from build123d import *

# Parameters (mm, degrees)
SKETCH1_W                   = 228.6
SKETCH1_H                   = 139.7
SKETCH1_W_2                 = 203.2
SKETCH1_H_2                 = 114.3
BOSS_EXTRUDE1_DEPTH         = 6.35
BOSS_EXTRUDE2_DEPTH         = 6.35
FILLET1_R                   = 6.35
FILLET2_R                   = 6.35
F_1_4_CLEARANCE_HOLE1_D     = 6.7564
F_1_4_CLEARANCE_HOLE1_DEPTH = 9.906
F_1_4_CLEARANCE_HOLE1_TIP   = 2.029827343


with BuildPart() as part:
    # Sketch1 → Boss-Extrude1 (new body)
    with BuildSketch(Plane.XY):
        Rectangle(SKETCH1_W, SKETCH1_H)
        Rectangle(SKETCH1_W_2, SKETCH1_H_2, mode=Mode.SUBTRACT)
    extrude(amount=BOSS_EXTRUDE1_DEPTH)

    # Sketch2 → Boss-Extrude2 (add)
    with BuildSketch(Plane.XY.offset(6.35)):
        with BuildLine():
            Line((-96.930261692, 65.451756991), (0, 10.928484789))
            Line((0, 10.928484789), (96.930261692, 65.451756991))
            ThreePointArc((96.930261692, 65.451756991), (109.901756991, 61.819738308), (106.269738308, 48.848243009))
            Line((106.269738308, 48.848243009), (19.428417403, 0))
            Line((19.428417403, 0), (106.269738308, -48.848243009))
            ThreePointArc((106.269738308, -48.848243009), (109.901756991, -61.819738308), (96.930261692, -65.451756991))
            Line((96.930261692, -65.451756991), (0, -10.928484789))
            Line((0, -10.928484789), (-96.930261692, -65.451756991))
            ThreePointArc((-96.930261692, -65.451756991), (-109.901756991, -61.819738308), (-106.269738308, -48.848243009))
            Line((-106.269738308, -48.848243009), (-19.428417403, 0))
            Line((-19.428417403, 0), (-106.269738308, 48.848243009))
            ThreePointArc((-106.269738308, 48.848243009), (-109.901756991, 61.819738308), (-96.930261692, 65.451756991))
        make_face()
    extrude(amount=-BOSS_EXTRUDE2_DEPTH)

    # Fillet1
    fillet1_edges = [part.edges().sort_by_distance(p)[0] for p in [
        (82.171582597, 57.15, 3.175),
        (-82.171582597, 57.15, 3.175),
        (101.6, -46.221515211, 3.175),
        (101.6, 46.221515211, 3.175),
        (-82.171582597, -57.15, 3.175),
        (82.171582597, -57.15, 3.175),
        (-101.6, 46.221515211, 3.175),
        (-101.6, -46.221515211, 3.175),
        (0, 10.928484789, 3.175),
        (19.428417403, 0, 3.175),
        (0, -10.928484789, 3.175),
        (-19.428417403, 0, 3.175),
    ]]
    fillet(fillet1_edges, radius=FILLET1_R)

    # Fillet2
    fillet2_edges = [part.edges().sort_by_distance(p)[0] for p in [
        (114.3, -69.85, 3.175),
        (-114.3, -69.85, 3.175),
        (-114.3, 69.85, 3.175),
        (114.3, 69.85, 3.175),
    ]]
    fillet(fillet2_edges, radius=FILLET2_R)

    # 1/4 Clearance Hole1
    with Locations(Plane.XY.offset(6.35)):
        with Locations((-101.6, 57.15), (101.6, 57.15), (-101.6, -57.15), (101.6, -57.15)):
            Hole(F_1_4_CLEARANCE_HOLE1_D / 2, depth=F_1_4_CLEARANCE_HOLE1_DEPTH)
            with Locations((0, 0, -(F_1_4_CLEARANCE_HOLE1_DEPTH + F_1_4_CLEARANCE_HOLE1_TIP / 2))):  # 118° drill point
                Cone(0, F_1_4_CLEARANCE_HOLE1_D / 2, F_1_4_CLEARANCE_HOLE1_TIP, mode=Mode.SUBTRACT)


solid = part.part
Geometry: final body of the model. Coordinates: model frame, mm. A direction names the side the tool comes from. Coordinates: 2 decimals unless noted, no trailing zeros. Order: outer loops, then holes, each group sorted by start corner. A loop starts at its lowest first (then second) coordinate and runs counter-clockwise, first axis right, second up. Notation, with made-up numbers: M -10,-6.75 L 11,-6.75 A25 cw 11,5.25 Z; hole C 16.5,2.25 d9. An arc over 180 degrees is marked long. One line per question, with ' | ' between items. Start each with the question number.
Item 1: Draft query along Y for faces 1 (the flat face through (-2, 69.85, 3)), 2 (the flat face through (114.3, -1, 3)), 3 (the cylindrical face through (-99.11, 59.433, 3.131)). Return one class per face: released by +Y, released by -Y, zero draft, split by the parting line, or undercut.
Item 2: Set-up query: faces 4 (the flat face through (-61.142, -23.464, 3.219)), 5 (the cylindrical face through (-112.49, 67.94, 3.22)). Return all of +Z, -Z, +X, -X, +Y, -Y with unobstructed straight access to the full face (end or side cutting, diameter ignored); none if empty.
Item 3: Ray query, probe 1 along X at (y, z) = (51.5, 3.75); probe 2 along Y at (x, z) = (-58.5, 3.5); probe 3 along Y at (x, z) = (-30, 3.5). Return the intervals inside material, ascending. Write a range as [from, to].
Item 4: Cut plane B-B, the plane y = -21. Return the cut outline in (x, z).
Item 5: Cut plane A-A, the plane x = -75.5. Return the cut outline in (y, z).
Item 6: Cut plane C-C, the plane z = 3.75. Count the separate pieces of the cut face and the enclosed holes in it, then the cut area to 3 significant figures.
Item 7: Cut plane D-D, the plane x = 38. Return the cut outline in (y, z).
A:
1) face 1: released by +Y | face 2: zero draft | face 3: undercut
2) face 4: +Z, -Z | face 5: +Z, -Z, -X, +Y
3) probe 1: x = [-114.3, -64.24], [64.24, 114.3] | probe 2: y = [-69.85, -57.12], [-43.83, -21.98], [21.98, 43.83], [57.12, 69.85] | probe 3: y = [-69.85, -57.15], [-27.8, -5.95], [5.95, 27.8], [57.15, 69.85]
4) outline: M -114.3,0 L -101.6,0 L -101.6,6.35 L -114.3,6.35 Z; M -56.76,0 L -17.9,0 L -17.9,6.35 L -56.76,6.35 Z; M 17.9,0 L 56.76,0 L 56.76,6.35 L 17.9,6.35 Z; M 101.6,0 L 114.3,0 L 114.3,6.35 L 101.6,6.35 Z
5) outline: M -69.85,0 L -31.54,0 L -31.54,6.35 L -69.85,6.35 Z; M 31.54,0 L 69.85,0 L 69.85,6.35 L 31.54,6.35 Z
6) separate pieces: 1 | enclosed holes: 8 | area: 17,100 mm2
7) outline: M -69.85,0 L -57.15,0 L -57.15,6.35 L -69.85,6.35 Z; M -32.3,0 L -10.45,0 L -10.45,6.35 L -32.3,6.35 Z; M 10.45,0 L 32.3,0 L 32.3,6.35 L 10.45,6.35 Z; M 57.15,0 L 69.85,0 L 69.85,6.35 L 57.15,6.35 Z
